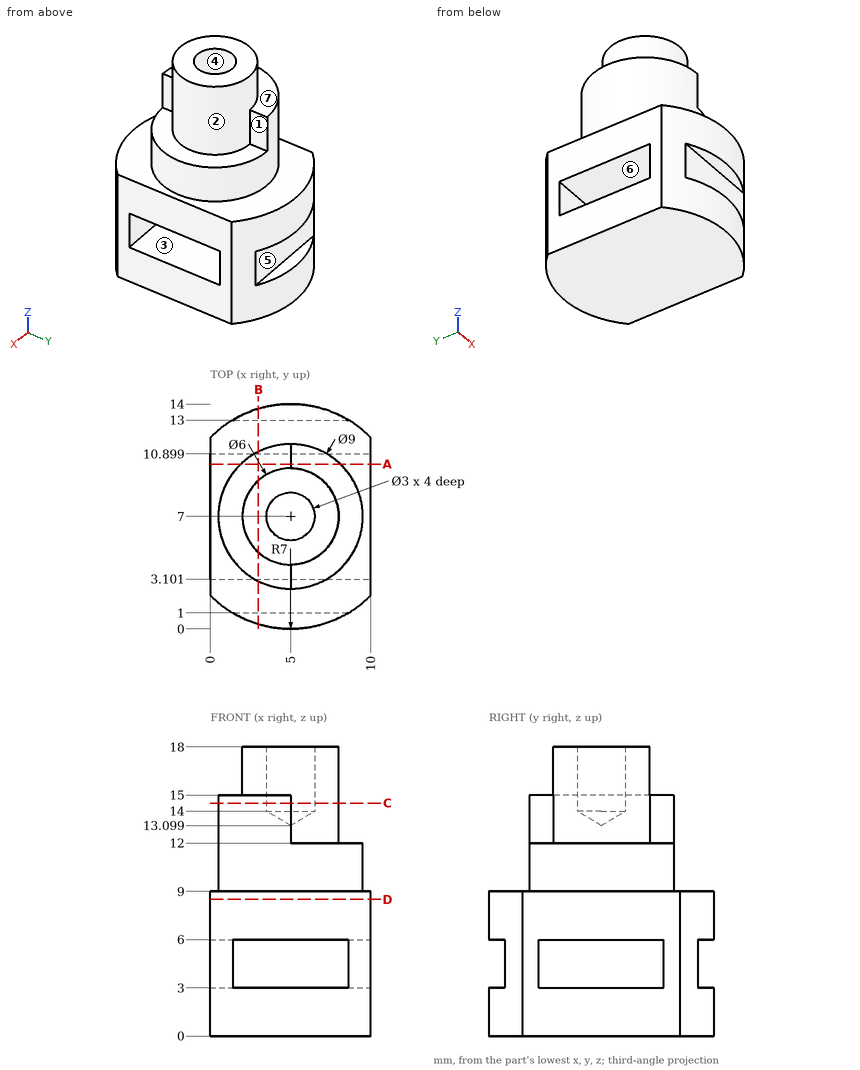
Input: dimensioned drawing with shaded views. Units: mm. Origin: part minimum x, y, z. A direction names the side the tool comes from. Give positions to 0.01 mm unless a question says otherwise; leave off trailing zeros. Order: outer loops, then holes, each group sorted by start corner. A loop starts at its lowest first (then second) coordinate and runs counter-clockwise, first axis right, second up. Notation, with made-up numbers: (-33.75, -20) -> (18.25, -20) arc R8 cw to (18.25, -7) -> close; hole circle Ø2 at (-21, -13.75). An arc over 180 degrees is marked (long way). Answer as a JSON object with one key per item and string values.
Q1. Section B-B (x = 3). Output: boundary loops of the cut face in (y, z).
Entries:
{"outline": "(0.29, 0) -> (13.71, 0) -> (13.71, 3) -> (13, 3) -> (13, 6) -> (13.71, 6) -> (13.71, 9) -> (11.03, 9) -> (11.03, 15) -> (9.24, 15) -> (9.24, 18) -> (4.76, 18) -> (4.76, 15) -> (2.97, 15) -> (2.97, 9) -> (0.29, 9) -> (0.29, 6) -> (1, 6) -> (1, 3) -> (0.29, 3) -> close; hole (3.1, 3) -> (10.9, 3) -> (10.9, 6) -> (3.1, 6) -> close"}
Q2. Material intervals for probe 1 along Y at (x, z) = (5, 16.5); probe 2 along Z at (x, y) = (7.5, 7.75); probe 3 along Z at (x, y) = (8, 3.5), sorted ascending.
Entries:
{"probe 1": "y = 4 to 5.5, 8.5 to 10", "probe 2": "z = 0 to 3, 6 to 18", "probe 3": "z = 0 to 3, 6 to 9"}
Q3. Access query for the marked faces 4, 5, 6 and 7. Directions: +Z, -Z, +X, -X, +Y, -Y. A direction counts if a zero-diameter tool reaches every point of the face in a straight line with its end or side. Return the directions, or none.
Entries:
{"face 4": "+Z", "face 5": "+X, -X, +Y", "face 6": "+X, -X", "face 7": "+Z, -X"}
Q4. Draft query along Y for the marked faces 1, 2 and 3. Return one class per face: released by +Y, released by -Y, zero draft, split by the parting line, or undercut.
Entries:
{"face 1": "zero draft", "face 2": "split by the parting line", "face 3": "undercut"}
Q5. Section A-A (y = 10.25). Output: boundary loops of the cut face in (x, z).
Entries:
{"outline": "(0, 0) -> (10, 0) -> (10, 3) -> (0, 3) -> close; (0, 6) -> (10, 6) -> (10, 9) -> (8.11, 9) -> (8.11, 12) -> (5, 12) -> (5, 15) -> (1.89, 15) -> (1.89, 9) -> (0, 9) -> close"}
Q6. Section D-D (z = 8.5). Output: boundary loops of the cut face in (x, y), plus the area to 3 significant figures.
Entries:
{"outline": "(0, 2.1) arc R7 ccw to (10, 2.1) -> (10, 11.9) arc R7 ccw to (0, 11.9) -> close", "area": "127 mm^2"}
Q7. Section C-C (z = 14.5). Output: boundary loops of the cut face in (x, y), plus the area to 3 significant figures.
Entries:
{"outline": "(5, 2.5) -> (5, 4) arc R3 ccw to (5, 10) -> (5, 11.5) arc R4.5 ccw to start; hole circle Ø3 at (5, 7)", "area": "38.9 mm^2"}
Q8. First-contact query: pin 1 (4 mm diameter, centred on x = 3, z = 12.5, fed in from +Y); pin 2 (2.5 mm diameter, centred on x = 4, z = 4.5, fed in from +Y); pin 3 (1.6 mm diameter, centred on y = 11, z = 14, fed in from +X). Flat tips, straight axial feed; report the tip coordinate or a pass-through.
Entries:
{"pin 1": "stops at y = 11.5", "pin 2": "stops at y = 13", "pin 3": "stops at x = 5"}
